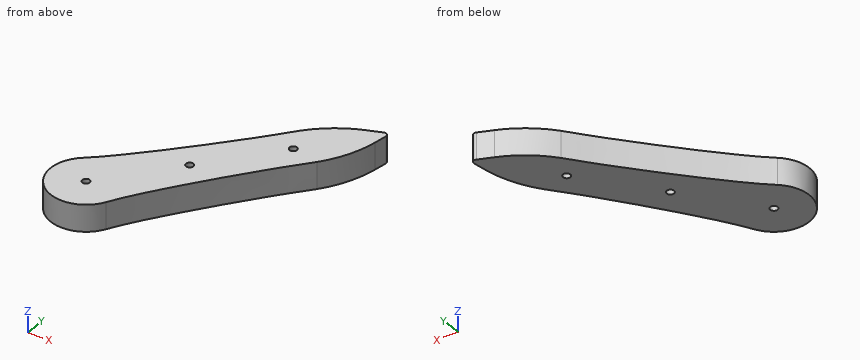
from build123d import *

# Parameters (mm, degrees)
SKETCH3_R           = 1.6
BOSS_EXTRUDE1_DEPTH = 15
CUT_EXTRUDE1_START  = -15
SKETCH4_R           = 1.6
CUT_EXTRUDE1_DEPTH  = 15
FILLET3_R           = 62
SKETCH5_R           = 2.1
CUT_EXTRUDE2_DEPTH  = 15
FILLET4_R           = 2


with BuildPart() as part:
    # Sketch3 → Boss-Extrude1 (new body)
    with BuildSketch(Plane.XY.offset(16)):
        with BuildLine():
            ThreePointArc((155.019115612, -142.985112199), (159.394881243, -97.849485606), (115.704809966, -109.996492831))
            add(Edge.make_bspline(
                [(115.704809966, -109.996492831), (101.94879758, -150.116707379), (78.178790791, -171.772825461), (58.717079478, -197.082387325), (16.356999542, -244.049515564), (0.72448619, -256.46124476)],
                knots=[0, 0, 0, 0, 0.619090324, 0.719090324, 1, 1, 1, 1], degree=3))
            ThreePointArc((0.72448619, -256.46124476), (0.304947846, -287.445485278), (30.74561606, -281.651963762))
            add(Edge.make_bspline(
                [(155.019115612, -142.985112199), (117.897123756, -163.498941991), (100.69762913, -190.668374405), (79.152067085, -214.229377889), (40.254225745, -264.101669257), (30.74561606, -281.651963762)],
                knots=[0, 0, 0, 0, 0.619090324, 0.719090324, 1, 1, 1, 1], degree=3))
        make_face()
        with Locations((135.218221977, -112.415707792)):
            Circle(SKETCH3_R, mode=Mode.SUBTRACT)
        with Locations((148.218221977, -112.415707792)):
            Circle(SKETCH3_R, mode=Mode.SUBTRACT)
        with Locations((148.218221977, -125.415707792)):
            Circle(SKETCH3_R, mode=Mode.SUBTRACT)
        with Locations((135.218221977, -125.415707792)):
            Circle(SKETCH3_R, mode=Mode.SUBTRACT)
        with Locations((77.439461008, -195.520152104)):
            Circle(SKETCH3_R, mode=Mode.SUBTRACT)
        with Locations((45.300080524, -233.82237426)):
            Circle(SKETCH3_R, mode=Mode.SUBTRACT)
        with Locations((13.16070004, -272.124596416)):
            Circle(SKETCH3_R, mode=Mode.SUBTRACT)
    extrude(amount=BOSS_EXTRUDE1_DEPTH)

    # Sketch4 → Cut-Extrude1 (cut)
    with BuildSketch(Plane.XY.offset(31).offset(CUT_EXTRUDE1_START)):
        with BuildLine():
            add(Edge.make_bspline(
                [(115.704809966, -109.996492831), (106.058622012, -138.130164086), (93.113701565, -155.703600822), (81.681620369, -169.238644056)],
                knots=[0, 0, 0, 0, 0.434127381, 0.434127381, 0.434127381, 0.434127381], degree=3))
            Line((81.681620369, -169.238644056), (107.801063948, -159.441089101))
            Line((107.801063948, -159.441089101), (103.173332299, -186.075062907))
            add(Edge.make_bspline(
                [(155.019115612, -142.985112199), (129.435323739, -157.122865204), (114.450199889, -172.627251292), (103.173332299, -186.075062907)],
                knots=[0, 0, 0, 0, 0.426665629, 0.426665629, 0.426665629, 0.426665629], degree=3))
            ThreePointArc((155.019115612, -142.985112199), (157.145110388, -141.681056767), (159.144213742, -140.189748569))
            Line((159.144213742, -140.189748569), (159.161693107, -140.175418866))
            ThreePointArc((159.161693107, -140.175418866), (158.677203155, -97.267544882), (116.900921238, -107.068700404))
            ThreePointArc((116.900921238, -107.068700404), (116.260741116, -108.51538721), (115.704809966, -109.996492831))
        make_face()
        with Locations((135.218221977, -125.415707792)):
            Circle(SKETCH4_R, mode=Mode.SUBTRACT)
        with Locations((148.218221977, -125.415707792)):
            Circle(SKETCH4_R, mode=Mode.SUBTRACT)
        with Locations((135.218221977, -112.415707792)):
            Circle(SKETCH4_R, mode=Mode.SUBTRACT)
        with Locations((148.218221977, -112.415707792)):
            Circle(SKETCH4_R, mode=Mode.SUBTRACT)
    extrude(amount=CUT_EXTRUDE1_DEPTH, mode=Mode.SUBTRACT)


with BuildPart() as cut_extrude1_kept_piece:
    # of the separate pieces the step leaves, the one the design keeps (cut_extrude1_pieces_kept)
    add(part.part.solids().sort_by_distance((30.74561606, -281.651963762, 16))[0])

    # Fillet3
    fillet3_edges = [cut_extrude1_kept_piece.edges().sort_by_distance(p)[0] for p in [
        (81.681620369, -169.238644056, 23.5),
        (103.173332299, -186.075062907, 23.5),
    ]]
    fillet(fillet3_edges, radius=FILLET3_R)

    # Sketch5 → Cut-Extrude2 (cut)
    with BuildSketch(Plane.XY.offset(31)):
        with Locations((77.439461008, -195.520152104)):
            Circle(SKETCH5_R)
        with Locations((45.300080524, -233.82237426)):
            Circle(SKETCH5_R)
        with Locations((13.16070004, -272.124596416)):
            Circle(SKETCH5_R)
    extrude(amount=-CUT_EXTRUDE2_DEPTH, mode=Mode.SUBTRACT)

    # Fillet4
    fillet4_edges = [cut_extrude1_kept_piece.edges().sort_by_distance(p)[0] for p in [
        (107.801063948, -159.441089101, 23.5),
    ]]
    fillet(fillet4_edges, radius=FILLET4_R)


solid = cut_extrude1_kept_piece.part
The model under review builds one solid part; all positions refer to its coordinate system, in mm. Coordinates: 2 decimals unless noted, no trailing zeros. Use a Markdown table: item, result. Add a question column.
1. Clearance check with flat-ended pins moving along their axes: pin 1 Ø2 at (y, z) = (-265.5, 28) entering from -X; pin 2 Ø6 at (y, z) = (-182.5, 22) entering from +X; pin 3 Ø8 at (x, z) = (69.5, 27.5) entering from -Y; pin 4 Ø3.5 at (x, y) = (45.3, -233.82) entering from -Z. State where each tip first meets the part, or that it passes through.
2. To check wall thickness, follow line 1 (Y direction, x = 76, z = 25.25); line 2 (Y direction, x = 67, z = 17.5); line 3 (Y direction, x = 19.5, z = 18.75). State the ranges of each line that lie inside material, in increasing order.
3. Add section A-A on z = 21. Give the number of separate pieces and of enclosed holes in the cut face, plus the area to 3 significant figures.
Returned:
| question | item | result |
|---|---|---|
| 1 | pin 1 | stops at x = -6.03 |
| 1 | pin 2 | stops at x = 103.54 |
| 1 | pin 3 | stops at y = -232.17 |
| 1 | pin 4 | passes through |
| 2 | line 1 | y = -218.86 to -197.05, -193.99 to -176.36 |
| 2 | line 2 | y = -230.24 to -186.4 |
| 2 | line 3 | y = -291.09 to -239 |
| 3 | separate pieces | 1 |
| 3 | enclosed holes | 3 |
| 3 | area | 4,640 mm² |
